Build history of the part. All positions in model axes, mm. A direction names the side the tool comes from. Round coordinates to 2 decimals unless told otherwise and drop trailing zeros. Write each loop counter-clockwise with the first axis right and the second up, starting at its lowest first coordinate (ties: lowest second). Pieces come first, ordered by that corner, then holes. Notation, with made-up numbers: (33, -36) -> (74, -36) arc R15 ccw to (74, -29) -> close; hole circle Ø4 at (38, -0.5). An arc over 180 degrees is marked (long way). Answer in a Markdown table with one row per item.
```python
from build123d import *

# Parameters (mm, degrees)
SKETCH_1_R          = 8
SKETCH_1_R_2        = 2
EXTRUDE_1_DEPTH     = 5
SKETCH_3_W          = 32
SKETCH_3_H          = 5.5
EXTRUDE_3_DEPTH     = 5
EXTRUDE_4_DEPTH     = 30
SKETCH_6_R          = 1.5
CUT_EXTRUDE_1_DEPTH = 20
SKETCH_7_W          = 3
SKETCH_7_H          = 8.5
CUT_EXTRUDE_5_DEPTH = 30


with BuildPart() as part:
    # 草图1 → 凸台-拉伸1 (new body)
    with BuildSketch(Plane(origin=(0, 0, 0), x_dir=(0, 0, -1), z_dir=(1, 0, 0))):
        with BuildLine():
            Line((-16, 0), (-16, -16))
            Line((-16, -16), (16, -16))
            Line((16, -16), (16, 0))
            ThreePointArc((16, 0), (0, 16), (-16, 0))
        make_face()
        Circle(SKETCH_1_R, mode=Mode.SUBTRACT)
        with Locations((-12, 0)):
            Circle(SKETCH_1_R_2, mode=Mode.SUBTRACT)
        with Locations((12, 0)):
            Circle(SKETCH_1_R_2, mode=Mode.SUBTRACT)
    extrude(amount=EXTRUDE_1_DEPTH)

    # 草图3 → 凸台-拉伸3 (add)
    with BuildSketch(Plane(origin=(5, 0, 0), x_dir=(0, 0, -1), z_dir=(1, 0, 0))):
        with Locations((0, -13.25)):
            Rectangle(SKETCH_3_W, SKETCH_3_H)
    extrude(amount=EXTRUDE_3_DEPTH)

    # 草图4 → 凸台-拉伸4 (add)
    with BuildSketch(Plane.ZY):
        with BuildLine():
            Line((-8, 4), (-15.491933385, 4))
            ThreePointArc((-15.491933385, 4), (-15.87247514, 2.01606868), (-16, 0))
            Line((-16, 0), (-16, -16))
            Line((-16, -16), (-3, -16))
            Line((-3, -16), (-3, -13))
            Line((-3, -13), (-8, -13))
            Line((-8, -13), (-8, 4))
        make_face()
        with BuildLine():
            Line((3, -13), (3, -16))
            Line((3, -16), (16, -16))
            Line((16, -16), (16, 0))
            ThreePointArc((16, 0), (15.87247514, 2.01606868), (15.491933385, 4))
            Line((15.491933385, 4), (8, 4))
            Line((8, 4), (8, -13))
            Line((8, -13), (3, -13))
        make_face()
    extrude(amount=EXTRUDE_4_DEPTH)

    # 草图6 → 切除-拉伸1 (cut)
    with BuildSketch(Plane(origin=(0, -13, 0), x_dir=(1, 0, 0), z_dir=(0, 1, 0))):
        with Locations((-6, -7.5)):
            Circle(SKETCH_6_R)
        with Locations((-6, 7.5)):
            Circle(SKETCH_6_R)
        with Locations((-26, 7.5)):
            Circle(SKETCH_6_R)
        with Locations((-26, -7.5)):
            Circle(SKETCH_6_R)
    extrude(amount=-CUT_EXTRUDE_1_DEPTH, mode=Mode.SUBTRACT)

    # 草图7 → 切除-拉伸5 (cut)
    with BuildSketch(Plane.ZY.offset(30)):
        with Locations((-9.5, -8.75)):
            Rectangle(SKETCH_7_W, SKETCH_7_H)
        with Locations((9.5, -8.75)):
            Rectangle(SKETCH_7_W, SKETCH_7_H)
    extrude(amount=-CUT_EXTRUDE_5_DEPTH, mode=Mode.SUBTRACT)


solid = part.part
```
Q1. Saw through at C-C on z = 7.5. Write the cut outline in (x, y), plus the area to 3 significant figures.
A:
| item | result |
|---|---|
| outline | (-30, -16) -> (-27.5, -16) -> (-27.5, -13) -> (-30, -13) -> close; (-24.5, -16) -> (-7.5, -16) -> (-7.5, -13) -> (-24.5, -13) -> close; (-4.5, -16) -> (10, -16) -> (10, -10.5) -> (5, -10.5) -> (5, -2.78) -> (0, -2.78) -> (0, -13) -> (-4.5, -13) -> close; (0, 2.78) -> (5, 2.78) -> (5, 14.13) -> (0, 14.13) -> close |
| area | 222 mm² |
Q2. Wall check: line 1 (Z direction, x = -26, y = -14.95); line 2 (Z direction, x = -25, y = -8.5); line 3 (Y direction, x = -7, z = -9). Give the ranges that are in metal, low to high. Write a range as [from, to].
A:
| item | result |
|---|---|
| line 1 | [-16, -9], [-6, -3], [3, 6], [9, 16] |
| line 2 | [-16, -11], [11, 16] |
| line 3 | [-16, -13], [-4.5, 4] |
Q3. Saw through at A-A on x = -23. Write the cut outline in (y, z), plus the area to 3 significant figures.
A:
| item | result |
|---|---|
| outline | (-16, -16) -> (0, -16) arc R16 ccw to (4, -15.49) -> (4, -8) -> (-4.5, -8) -> (-4.5, -11) -> (-13, -11) -> (-13, -3) -> (-16, -3) -> close; (-16, 3) -> (-13, 3) -> (-13, 11) -> (-4.5, 11) -> (-4.5, 8) -> (4, 8) -> (4, 15.49) arc R16 ccw to (0, 16) -> (-16, 16) -> close |
| area | 298 mm² |
Q4. Drop flat-ended pins along their axis: P1, Ø8, axis at y = 2, z = 8, coming from the +X side; P2, Ø9, axis at x = -20, z = -8, coming from the +Y side; P3, Ø2, axis at x = -3.5, z = 5.5, coming from the +Y side; P4, Ø1.5, axis at x = -9, y = 5.5, coming from the +Z side. Give the stop position or say it passes through.
A:
| item | result |
|---|---|
| P1 | x = 5 |
| P2 | y = 4 |
| P3 | y = -13 |
| P4 | through |
Q5. Saw through at D-D on y = -4. Write the cut outline in (x, z), plus the area to 3 significant figures.
A:
| item | result |
|---|---|
| outline | (-30, -16) -> (5, -16) -> (5, -6.93) -> (0, -6.93) -> (0, -8) -> (-30, -8) -> close; (-30, 8) -> (0, 8) -> (0, 6.93) -> (5, 6.93) -> (5, 16) -> (-30, 16) -> close |
| area | 571 mm² |
Q6. Saw through at B-B on x = -6. Write the cut outline in (y, z), plus the area to 3 significant figures.
A:
| item | result |
|---|---|
| outline | (-16, -16) -> (0, -16) arc R16 ccw to (4, -15.49) -> (4, -8) -> (-4.5, -8) -> (-4.5, -11) -> (-13, -11) -> (-13, -9) -> (-16, -9) -> close; (-16, -6) -> (-13, -6) -> (-13, -3) -> (-16, -3) -> close; (-16, 3) -> (-13, 3) -> (-13, 6) -> (-16, 6) -> close; (-16, 9) -> (-13, 9) -> (-13, 11) -> (-4.5, 11) -> (-4.5, 8) -> (4, 8) -> (4, 15.49) arc R16 ccw to (0, 16) -> (-16, 16) -> close |
| area | 280 mm² |
Q7. Two-plate mould, pull along Y, no slides. Class faces 4 (the flat face through (-15, 0, -8)), 5 (the flat face through (-15, 4, -12)), 6 (the flat face through (-15, -13, -7)), 7 (the cylindrical face through (2.5, -1.2, 13.6)): released by +Y, released by -Y, zero draft, split by the parting line, or undercut.
A:
| item | result |
|---|---|
| face 4 | zero draft |
| face 5 | released by +Y |
| face 6 | undercut |
| face 7 | undercut |
Q8. Which spindle directions (+Z, -Z, +X, -X, +Y, -Y) get a long thin tool onto all of the face, cutting with end or side? Do faces 1 (the cylindrical face through (-6, -14, 9)), 2 (the flat face through (-15, 0, 8)), 3 (the flat face through (-15, -9, 11)). Say none if no direction does.
A:
| item | result |
|---|---|
| face 1 | -Y |
| face 2 | -X, +Y |
| face 3 | -X |
